Verification items for the finished model (mm, model axes). Give positions to 0.01 mm unless a question says otherwise; leave off trailing zeros. Order: outer loops, then holes, each group sorted by start corner. A loop starts at its lowest first (then second) coordinate and runs counter-clockwise, first axis right, second up.
(1) Gauge pin test, flat end, axial feed: pin 1 (17 mm diameter, centred on y = -85.725, z = -9.525, fed in from +X). Record the tip position at first contact, or that the pin passes through.
(2) Sectioned sample at B-B on z = 9. Record the cut outline in (x, y) (3 decimals), plus the area to 3 significant figures.
(3) Sectioned sample at D-D on y = -42.5. Record the cut outline in (x, z), plus the area to 3 significant figures.
(4) Sectioned sample at C-C on x = 2.75. Record the cut outline in (y, z) (3 decimals), plus the area to 3 significant figures.
(5) Sectioned sample at A-A on y = 0. Record the cut outline in (x, z) (3 decimals).
(6) Scan lines: L1, parallel to Z at x = 2.5, y = 0 (3 decimals); L2, parallel to Y at x = 5.75, z = 3.5 (3 decimals); L3, parallel to Y at x = 5.25, z = -16. Record each from-to range of solid material in increasing order.
```python
from build123d import *

# Parameters (mm, degrees)
F0_R     = 9.525
F0_W     = 139.7
F0_H     = 38.1
F0_R_2   = 3.175
F1_DEPTH = 6.35


with BuildPart() as f1:
    # F0 (on Right) → F1 (new body)
    with BuildSketch(Plane.YZ):
        with BuildLine():
            Line((-85.725, -25.4), (85.725, -25.4))
            ThreePointArc((85.725, -25.4), (94.705256, -21.680256), (98.425, -12.7))
            Line((98.425, -12.7), (98.425, 17.298685))
            ThreePointArc((98.425, 17.298685), (96.432049, 24.128699), (91.078686, 28.81511))
            Line((91.078686, 28.81511), (5.353686, 68.666425))
            ThreePointArc((5.353686, 68.666425), (0, 69.85), (-5.353686, 68.666425))
            Line((-5.353686, 68.666425), (-91.078686, 28.81511))
            ThreePointArc((-91.078686, 28.81511), (-96.432049, 24.128699), (-98.425, 17.298685))
            Line((-98.425, 17.298685), (-98.425, -12.7))
            ThreePointArc((-98.425, -12.7), (-94.705256, -21.680256), (-85.725, -25.4))
        make_face()
        with Locations((-85.725, -9.525)):
            Circle(F0_R, mode=Mode.SUBTRACT)
        with Locations((85.725, -9.525)):
            Circle(F0_R, mode=Mode.SUBTRACT)
        Rectangle(F0_W, F0_H, mode=Mode.SUBTRACT)
        with Locations((0, 63.5)):
            Circle(F0_R_2, mode=Mode.SUBTRACT)
    extrude(amount=F1_DEPTH)


solid = f1.part
```
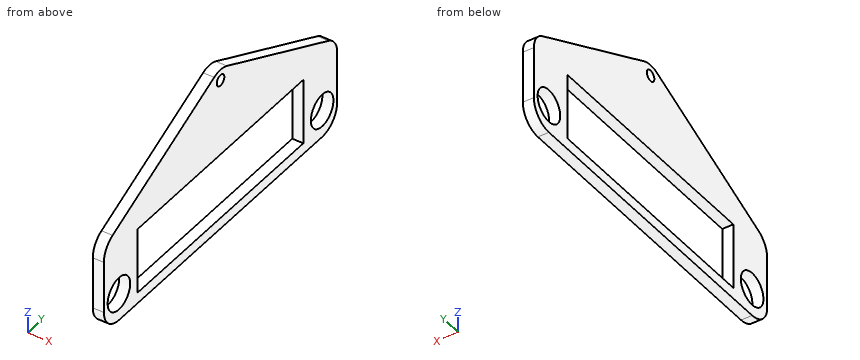
Ans:
1. pin 1: passes through
2. outline: (0, -98.425) - (6.35, -98.425) - (6.35, -69.85) - (0, -69.85) - close; (0, 69.85) - (6.35, 69.85) - (6.35, 98.425) - (0, 98.425) - close
2. area: 363 mm2
3. outline: (0, -25.4) - (6.35, -25.4) - (6.35, -19.05) - (0, -19.05) - close; (0, 19.05) - (6.35, 19.05) - (6.35, 51.4) - (0, 51.4) - close
3. area: 246 mm2
4. outline: (-98.425, -12.7) arc R12.7 ccw to (-85.725, -25.4) - (85.725, -25.4) arc R12.7 ccw to (98.425, -12.7) - (98.425, 17.299) arc R12.7 ccw to (91.079, 28.815) - (5.354, 68.666) arc R12.7 ccw to (-5.354, 68.666) - (-91.079, 28.815) arc R12.7 ccw to (-98.425, 17.299) - close; hole circle Ø19.05 at (-85.725, -9.525); hole (-69.85, -19.05) - (69.85, -19.05) - (69.85, 19.05) - (-69.85, 19.05) - close; hole circle Ø6.35 at (0, 63.5); hole circle Ø19.05 at (85.725, -9.525)
4. area: 8,480 mm2
5. outline: (0, -25.4) - (6.35, -25.4) - (6.35, -19.05) - (0, -19.05) - close; (0, 19.05) - (6.35, 19.05) - (6.35, 60.325) - (0, 60.325) - close; (0, 66.675) - (6.35, 66.675) - (6.35, 69.85) - (0, 69.85) - close
6. L1: z = -25.4 to -19.05, 19.05 to 60.325, 66.675 to 69.85
6. L2: y = -98.425 to -69.85, 69.85 to 98.425
6. L3: y = -97.99 to -92.71, -78.74 to -69.85, 69.85 to 78.74, 92.71 to 97.99
